Can you work these out from the drawing? Everything is in mm from the part's minimum corner. Round coordinates to 2 decimals unless told otherwise and drop trailing zeros. Write each loop counter-clockwise with the first axis right and the second up, starting at its lowest first coordinate (ties: lowest second). Pieces come first, ordered by that corner, then holes. Notation, with made-up numbers: (-6, 19) - (14, 19) arc R14 ccw to (14, 46) - close; hole circle Ø7 at (-35, 7). An arc over 180 degrees is marked (long way). One line per item, written item: value. Start each with the question number.
(1) I'm going to push flat-ended pins straight in: pin 1 Ø1.5 at (y, z) = (3.5, 34) entering from -X; pin 2 Ø12 at (x, z) = (55, 13) entering from -Y. Where does each tip first touch, or does it pass through?
(2) I want a section at C-C on y = 1.8. List the corners of the cut face in (x, z) for me (1 decimal).
(3) I want a section at D-D on z = 38.5. List the corners of the cut face in (x, y) for me (1 decimal).
(4) I want a section at A-A on x = 31.5. List the corners of the cut face in (y, z) for me (1 decimal).
(5) I want a section at B-B on z = 15. List the corners of the cut face in (x, y) for me.
(6) If I drill on L1, parallel to X at y = 3.35, z = 31.5 (1 decimal); L2, parallel to Y at x = 55.5, z = 18.5; L3, parallel to X at y = 3.7, z = 39 (1 decimal), over which ranges is the centre line in solid material (lowest first)? Write a range as from..to.
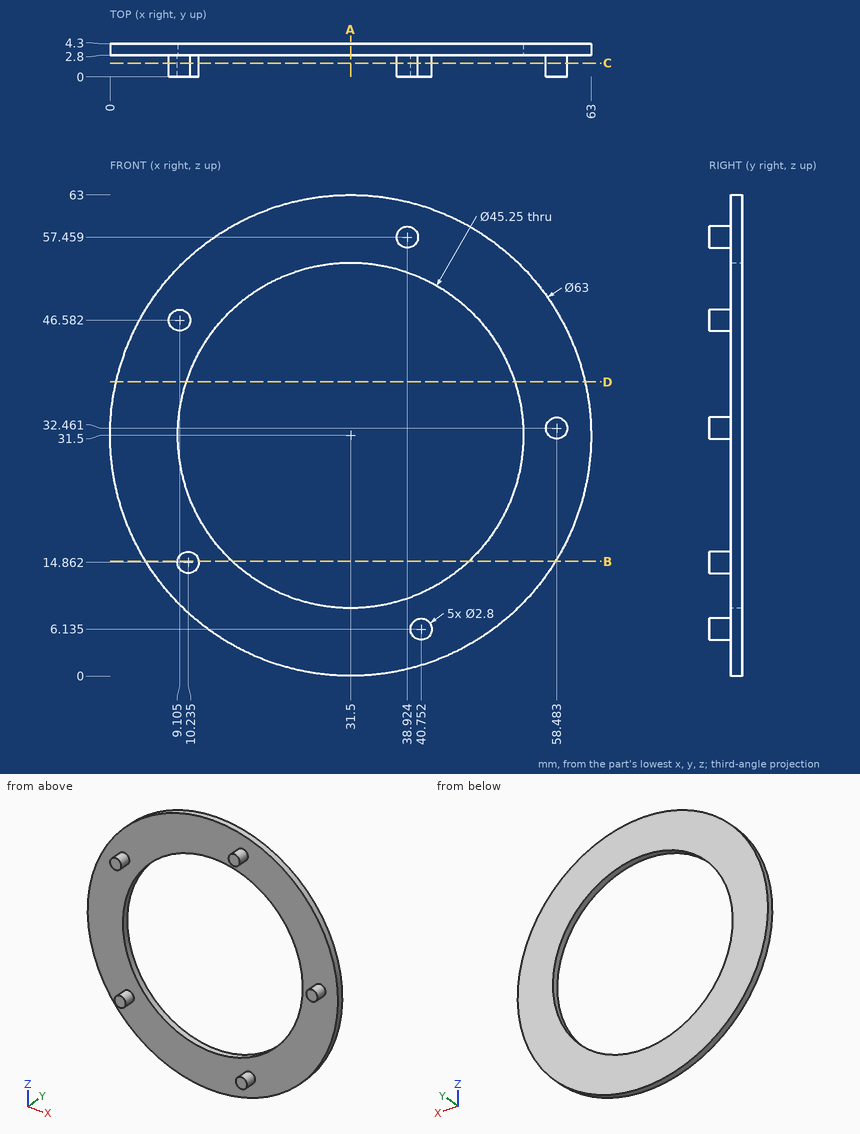
Established:
1. pin 1: x = 0.05
1. pin 2: y = 2.8
2. outline: circle Ø2.8 at (9.1, 46.6); circle Ø2.8 at (10.2, 14.9); circle Ø2.8 at (38.9, 57.5); circle Ø2.8 at (40.8, 6.1); circle Ø2.8 at (58.5, 32.5)
3. outline: (0.8, 2.8) - (10, 2.8) - (10, 4.3) - (0.8, 4.3) - close; (53, 2.8) - (62.2, 2.8) - (62.2, 4.3) - (53, 4.3) - close
4. outline: (2.8, 0) - (4.3, 0) - (4.3, 8.9) - (2.8, 8.9) - close; (2.8, 54.1) - (4.3, 54.1) - (4.3, 63) - (2.8, 63) - close
5. outline: (4.67, 2.8) - (8.84, 2.8) - (8.84, 0) - (11.63, 0) - (11.63, 2.8) - (16.02, 2.8) - (16.02, 4.3) - (4.67, 4.3) - close; (46.98, 2.8) - (58.33, 2.8) - (58.33, 4.3) - (46.98, 4.3) - close
6. L1: 0..8.9, 54.1..63
6. L2: 2.8..4.3
6. L3: 0.9..10.2, 52.8..62.1
